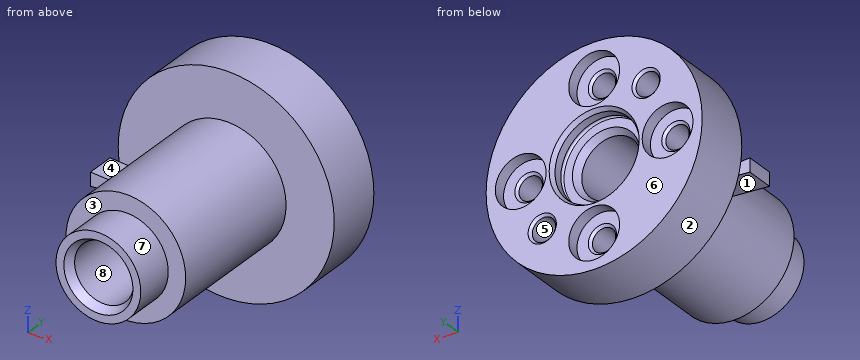
from build123d import *

# Parameters (mm, degrees)
SKETCH2_W                = 17.125
SKETCH2_H                = 5
REVOLVE2_ANGLE           = 4
REVOLVE2_OTHER_WAY_ANGLE = 4


with BuildPart() as part:
    # Sketch1 → Revolve1 (revolve)
    with BuildSketch(Plane.XY):
        Polygon((0, 42.7), (19.125, 42.7), (19.125, 32.6), (10.6, 32.6), (10.6, 7), (7.5, 7), (7.5, 0), (0, 0), align=None)
    revolve(axis=Axis((0, 0, 0), (0, 1, 0)))

    # Sketch2 → Revolve2 (revolve)
    with BuildSketch(Plane(origin=(0, 0, 0), x_dir=(-1, 0, 0), z_dir=(0, 0, -1))):
        with Locations((8.5625, 25.1)):
            Rectangle(SKETCH2_W, SKETCH2_H)
    revolve(axis=Axis((0, 22.6, 0), (0, 1, 0)), revolution_arc=REVOLVE2_ANGLE)

    # Sketch2 → Revolve2 other way (revolve)
    with BuildSketch(Plane(origin=(0, 0, 0), x_dir=(-1, 0, 0), z_dir=(0, 0, -1))):
        with Locations((8.5625, 25.1)):
            Rectangle(SKETCH2_W, SKETCH2_H)
    revolve(axis=Axis((0, 22.6, 0), (0, -1, 0)), revolution_arc=REVOLVE2_OTHER_WAY_ANGLE)

    # Sketch3 → Cut-Revolve1 (revolve, cut)
    with BuildSketch(Plane.XY):
        with BuildLine():
            Line((0, 42.7), (7.965, 42.7))
            Line((7.965, 42.7), (7.5, 41.894596374))
            Line((7.5, 41.894596374), (7.5, 40.4))
            ThreePointArc((7.5, 40.4), (7.8, 40), (7.5, 39.6))
            Line((7.5, 39.6), (6.00055535, 39.6))
            Line((6.00055535, 39.6), (5.25, 38.3))
            Line((5.25, 38.3), (5.25, 1.5))
            Line((5.25, 1.5), (6.116025404, 0))
            Line((6.116025404, 0), (0, 0))
            Line((0, 0), (0, 42.7))
        make_face()
    revolve(axis=Axis((0, 0, 0), (0, 1, 0)), mode=Mode.SUBTRACT)

    # Sketch4 → Cut-Revolve2 (revolve, cut)
    with BuildSketch(Plane.XY):
        Polygon((13, 42.7), (17.5, 42.7), (17.5, 40.6), (15.5, 40.6), (15.067, 40.167), (15.067, 34.6), (13, 33.406616994), align=None)
    revolve(axis=Axis((13, 33.406616994, 0), (0, 1, 0)), mode=Mode.SUBTRACT)

    # Sketch5 → Cut-Revolve3 (revolve, cut)
    with BuildSketch(Plane.XY):
        Polygon((-13, 42.7), (-8.5, 42.7), (-8.5, 40.6), (-10.5, 40.6), (-10.933, 40.167), (-10.933, 34.6), (-13, 33.406616994), align=None)
    revolve(axis=Axis((-13, 33.406616994, 0), (0, 1, 0)), mode=Mode.SUBTRACT)

    # Sketch6 → Cut-Revolve4 (revolve, cut)
    with BuildSketch(Plane(origin=(0, 0, 0), x_dir=(0, 0, -1), z_dir=(1, 0, 0))):
        Polygon((13, 42.7), (17.5, 42.7), (17.5, 40.6), (15.5, 40.6), (15.067, 40.167), (15.067, 34.6), (13, 33.406616994), align=None)
    revolve(axis=Axis((0, 33.406616994, -13), (0, 1, 0)), mode=Mode.SUBTRACT)

    # Sketch7 → Cut-Revolve5 (revolve, cut)
    with BuildSketch(Plane(origin=(0, 0, 0), x_dir=(0, 0, -1), z_dir=(1, 0, 0))):
        Polygon((-13, 42.7), (-8.5, 42.7), (-8.5, 40.6), (-10.5, 40.6), (-10.933, 40.167), (-10.933, 34.6), (-13, 33.406616994), align=None)
    revolve(axis=Axis((0, 33.406616994, 13), (0, 1, 0)), mode=Mode.SUBTRACT)

    # Sketch8 → Cut-Revolve6 (revolve, cut)
    with BuildSketch(Plane(origin=(0, 0, 0), x_dir=(0.707106781, 0, -0.707106781), z_dir=(0.707106781, 0, 0.707106781))):
        Polygon((13, 42.7), (15.5, 42.7), (15.067, 42.267), (15.067, 34.6), (13, 33.406616994), align=None)
    revolve(axis=Axis((9.192388155, 33.406616994, -9.192388155), (0, 1, 0)), mode=Mode.SUBTRACT)

    # Sketch9 → Cut-Revolve7 (revolve, cut)
    with BuildSketch(Plane(origin=(0, 0, 0), x_dir=(0.707106781, 0, -0.707106781), z_dir=(0.707106781, 0, 0.707106781))):
        Polygon((-13, 42.7), (-10.5, 42.7), (-10.933, 42.267), (-10.933, 34.6), (-13, 33.406616994), align=None)
    revolve(axis=Axis((-9.192388155, 33.406616994, 9.192388155), (0, 1, 0)), mode=Mode.SUBTRACT)


solid = part.part
Here's how the part is built. I have some questions about the finished solid (model axes, mm). Face numbers are marked on the shaded views. A direction names the side the tool comes from. Coordinates: 2 decimals unless noted, no trailing zeros. Loops run counter-clockwise (first coordinate to the right, second up) from the corner with the lowest first, then second, coordinate; pieces in that order, holes last. Notation, with made-up numbers: (-3, 54.5) -> (15, 54.5) arc R30 ccw to (15, 92.5) -> close; hole circle Ø5 at (72, 27). An arc over 180 degrees is marked (long way). Use one line per item in the form item = value. Start each with the question number.
(1) If we section it at A-A (y = 34): Please give me the cut outline in (x, z) (3 decimals).
(2) Will these pins go through, and if not, where does the flat tip stop? pin 1 (6.5 mm diameter, centred on x = -9.19, z = 9.19, fed in from -Y); pin 2 (3 mm diameter, centred on x = 10.5, y = 22.5, fed in from -Z); pin 3 (1.5 mm diameter, centred on y = 37.5, z = -4, fed in from +X).
(3) We'd pull the mould along X, two halves only. Please class the marked faces 1, 2 and 3: pulls with the +X half, pulls with the -X half, needs draft (parallel to the pull), parting line crosses it, or undercut.
(4) If we section it at B-B (y = 18.5): Please give me the cut outline in (x, z), then the cut area to 3 significant figures.
(5) On a 3-axis mill with a long thin cutter (end or side, diameter ignored), from which of +Z, -Z, +X, -X, +Y, -Y can I reach the whole of each face in a straight line? I mean the marked faces 4, 5, 6, 7 and 8. Say none if no direction works.
(6) Please list where these lines run through material, in increasing order: line 1 along Z through (x, y) = (0, 40.85) (3 decimals); line 2 along X through (y, z) = (22, 0); line 3 along X through (y, z) = (27.5, 0) (3 decimals).
Verdict:
q1.outline = circle Ø38.25 at (0, 0); hole circle Ø2.056 at (-13, 0); hole circle Ø2.056 at (-9.192, 9.192); hole circle Ø10.5 at (0, 0); hole circle Ø2.056 at (0, -13); hole circle Ø2.056 at (0, 13); hole circle Ø2.056 at (9.192, -9.192); hole circle Ø2.056 at (13, 0)
q2.pin_1 = 7
q2.pin_2 = -5.6
q2.pin_3 = 18.85
q3.face_1 = undercut
q3.face_2 = parting line crosses it
q3.face_3 = needs draft
q4.outline = circle Ø21.2 at (0, 0); hole circle Ø10.5 at (0, 0)
q4.area = 266 mm²
q5.face_4 = +Z, -Y
q5.face_5 = +Y
q5.face_6 = +Z, -Z, +X, -X, +Y
q5.face_7 = -Y
q5.face_8 = +Y, -Y
q6.line_1 = -19.125 to -17.5, -8.5 to -7.5, 7.5 to 8.5, 17.5 to 19.125
q6.line_2 = -10.6 to -5.25, 5.25 to 10.6
q6.line_3 = -17.125 to -5.25, 5.25 to 10.6
